CAD build for the part. Positions are in the model's coordinates, mm. Coordinates: 2 decimals unless noted, no trailing zeros. Write each loop counter-clockwise with the first axis right and the second up, starting at its lowest first coordinate (ties: lowest second). Pieces come first, ordered by that corner, then holes. Notation, with made-up numbers: (5.25, -15.75) - (27.25, -15.75) arc R32 cw to (27.25, 18.25) - close; hole circle Ø10 at (87, -5). An arc over 180 degrees is marked (long way). One line per question, with ' | ' between items. Start each with the question number.
1. Probe line 1 (Z direction, x = 2.5, y = 5); line 2 (Y direction, x = 2.75, z = 6); line 3 (X direction, y = 8, z = 1.25). List the from-to ranges inside material, lowest first.
2. Band-saw the part on A-A, the plane x = 0. Write the cut outline in (y, z) (3 decimals).
3. Band-saw the part on D-D, the plane z = 4. Write the cut outline in (x, y) (3 decimals), then the cut area to 3 significant figures.
4. Two-plate mould, pull along Z, no slides. Class faces 1 (the flat face through (0, 0, 0)), 2 (the cylindrical face through (-1.4, 10.66, 1.48)), 3 (the flat face through (0, 0, 9.5)): +Z half, -Z half, draft (parallel to the pull), parting line (faces both ways), or undercut.
5. Band-saw the part on C-C, the plane z = 2.25. Write the cut outline in (x, y), then the cut area to 3 significant figures.
6. Flat gauge pins, fed straight in: P1, Ø1.5, axis at x = -3.5, z = 4.5, coming from the +Y side; P2, Ø6, axis at x = -0.5, y = 8, coming from the +Z side; P3, Ø3, axis at x = 3.5, z = 6.5, coming from the -Y side. Where does each tip first touch, or does it go through?
from build123d import *

# Parameters (mm, degrees)
F0_R     = 10.75
F1_DEPTH = 3
F2_R     = 3.875
F3_DEPTH = 6.5
F4_SIZE2 = 5
F4_SIZE  = 0.25


with BuildPart() as f1:
    # F0 (on Top) → F1 (new body)
    with BuildSketch(Plane.XY):
        Circle(F0_R)
    extrude(amount=F1_DEPTH)

    # F2 (on face) → F3 (join)
    with BuildSketch(Plane.XY.offset(3)):
        Circle(F2_R)
    extrude(amount=F3_DEPTH)

    # F4
    f4_edges = [f1.edges().sort_by_distance(p)[0] for p in [
        (-3.875, 0, 9.5),
    ]]
    f4_side = f1.faces().sort_by_distance((0, 0, 9.5))[0]
    chamfer(f4_edges, length=F4_SIZE, length2=F4_SIZE2, reference=f4_side)


solid = f1.part
Filled in:
1) line 1: z = 0 to 3 | line 2: y = -2.62 to 2.62 | line 3: x = -7.18 to 7.18
2) outline: (-10.75, 0) - (10.75, 0) - (10.75, 3) - (3.875, 3) - (3.875, 4.5) - (3.625, 9.5) - (-3.625, 9.5) - (-3.875, 4.5) - (-3.875, 3) - (-10.75, 3) - close
3) outline: circle Ø7.75 at (0, 0) | area: 47.2 mm²
4) face 1: -Z half | face 2: draft | face 3: +Z half
5) outline: circle Ø21.5 at (0, 0) | area: 363 mm²
6) P1: stops at y = 2.73 | P2: stops at z = 3 | P3: stops at y = -3.21
